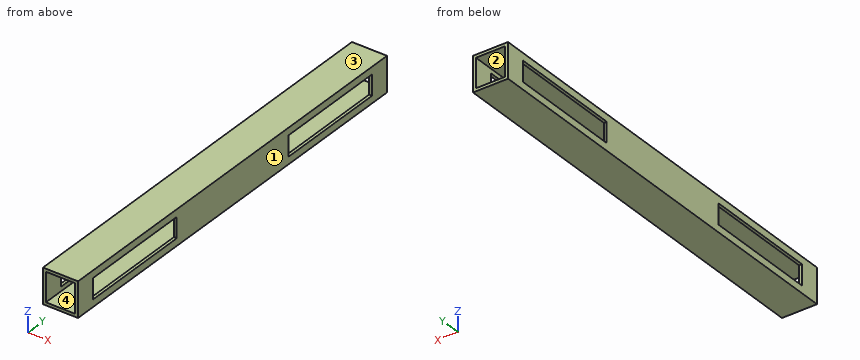
```python
from build123d import *

# Parameters (mm, degrees)
F0_W     = 76.2
F0_H     = 76.2
F0_W_2   = 63.5
F0_H_2   = 63.5
F1_DEPTH = 914.4
F2_W     = 247.65
F2_H     = 44.45
F3_DEPTH = 76.201


with BuildPart() as f1:
    # F0 (on Front) → F1 (new body)
    with BuildSketch(Plane.XZ):
        Rectangle(F0_W, F0_H)
        Rectangle(F0_W_2, F0_H_2, mode=Mode.SUBTRACT)
    extrude(amount=-F1_DEPTH)

    # F2 (on face) → F3 (cut, through all)
    with BuildSketch(Plane.YZ.offset(38.1)):
        with Locations((168.275, 0)):
            Rectangle(F2_W, F2_H)
        with Locations((746.125, 0)):
            Rectangle(F2_W, F2_H)
    extrude(amount=-F3_DEPTH, mode=Mode.SUBTRACT)


solid = f1.part
```
The model under review builds one solid part; all positions refer to its coordinate system, in mm. Face numbers are marked on the shaded views. Round coordinates to 2 decimals unless told otherwise and drop trailing zeros. Loops run counter-clockwise (first coordinate to the right, second up) from the corner with the lowest first, then second, coordinate; pieces in that order, holes last. Notation, with made-up numbers: (87, -23) -> (125, -23) arc R28 cw to (125, 12) -> close; hole circle Ø3 at (11, 16.25). An arc over 180 degrees is marked (long way). Answer in a Markdown table with one row per item.
1) Consider section B-B, the plane z = 5. Write out the cut boundary in (x, y), plus the area to 3 significant figures.
Taken from the geometry:
| item | result |
|---|---|
| outline | (-38.1, 0) -> (-31.75, 0) -> (-31.75, 44.45) -> (-38.1, 44.45) -> close; (-38.1, 292.1) -> (-31.75, 292.1) -> (-31.75, 622.3) -> (-38.1, 622.3) -> close; (-38.1, 869.95) -> (-31.75, 869.95) -> (-31.75, 914.4) -> (-38.1, 914.4) -> close; (31.75, 0) -> (38.1, 0) -> (38.1, 44.45) -> (31.75, 44.45) -> close; (31.75, 292.1) -> (38.1, 292.1) -> (38.1, 622.3) -> (31.75, 622.3) -> close; (31.75, 869.95) -> (38.1, 869.95) -> (38.1, 914.4) -> (31.75, 914.4) -> close |
| area | 5,320 mm² |
2) Draft analysis for pull direction X (two halves, no side actions). For the marked faces 1, 2, 3 and 4, state which applies: pulls with the +X half, pulls with the -X half, needs draft (parallel to the pull), parting line crosses it, or undercut.
Taken from the geometry:
| item | result |
|---|---|
| face 1 | pulls with the +X half |
| face 2 | undercut |
| face 3 | needs draft |
| face 4 | undercut |
3) For pin 1 Ø3 at (x, z) = (33.5, 4) entering from -Y, flat-tipped, find the tip position at first contact; note if it passes through.
Taken from the geometry:
| item | result |
|---|---|
| pin 1 | stops at y = 0 |
4) Wall thickness on line 1 along Z through (x, y) = (31, 244.5); line 2 along Z through (x, y) = (-32, 818.5) (3 decimals): over which ranges is each line inside the solid? List them lowest first.
Taken from the geometry:
| item | result |
|---|---|
| line 1 | z = -38.1 to -31.75, 31.75 to 38.1 |
| line 2 | z = -38.1 to -22.225, 22.225 to 38.1 |
5) Consider section C-C, the plane x = 14. Write out the cut boundary in (y, z), plus the area to 3 significant figures.
Taken from the geometry:
| item | result |
|---|---|
| outline | (0, -38.1) -> (914.4, -38.1) -> (914.4, -31.75) -> (0, -31.75) -> close; (0, 31.75) -> (914.4, 31.75) -> (914.4, 38.1) -> (0, 38.1) -> close |
| area | 11,600 mm² |
6) Consider section A-A, the plane y = 666. Write out the cut boundary in (x, z) (3 decimals).
Taken from the geometry:
| item | result |
|---|---|
| outline | (-38.1, -38.1) -> (38.1, -38.1) -> (38.1, -22.225) -> (31.75, -22.225) -> (31.75, -31.75) -> (-31.75, -31.75) -> (-31.75, -22.225) -> (-38.1, -22.225) -> close; (-38.1, 22.225) -> (-31.75, 22.225) -> (-31.75, 31.75) -> (31.75, 31.75) -> (31.75, 22.225) -> (38.1, 22.225) -> (38.1, 38.1) -> (-38.1, 38.1) -> close |
7) Consider section D-D, the plane y = 569. Write out the cut boundary in (x, z), plus the area to 3 significant figures.
Taken from the geometry:
| item | result |
|---|---|
| outline | (-38.1, -38.1) -> (38.1, -38.1) -> (38.1, 38.1) -> (-38.1, 38.1) -> close; hole (-31.75, -31.75) -> (31.75, -31.75) -> (31.75, 31.75) -> (-31.75, 31.75) -> close |
| area | 1,770 mm² |
